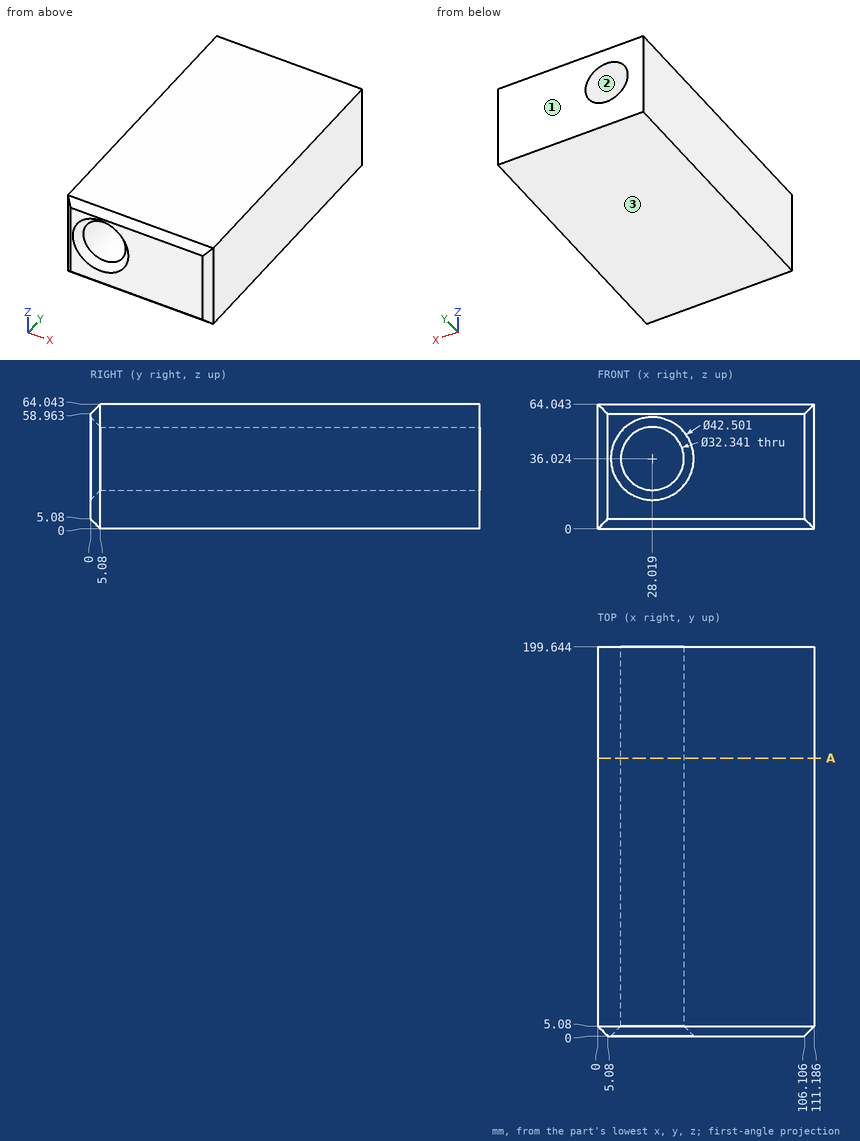
Geometry check sheet. Reference: drawing and pictorial views, mm from the part's lowest x, y, z. Coordinates: 2 decimals unless noted, no trailing zeros. Write each loop counter-clockwise with the first axis right and the second up, starting at its lowest first coordinate (ties: lowest second). Pieces come first, ordered by that corner, then holes. Notation, with made-up numbers: (9.5, 69.25) - (26.5, 69.25) arc R20 cw to (26.5, 98.25) - close; hole circle Ø3 at (50, 28). An arc over 180 degrees is marked (long way). Write item = value, one per line.
Q1. Go/stop test with a flat-tipped pin: pin 1 Ø12 at (x, y) = (59.5, 103.5) entering from -Z. Record where the tip stops, or that it passes through.
Answer:
pin_1 = 0
Q2. Mould release check, pull along Z, two halves, no side actions. Record for the marked faces 1, 2 and 3: released by +Z, released by -Z, zero draft, split by the parting line, or undercut.
Answer:
face_1 = zero draft
face_2 = undercut
face_3 = released by -Z
Q3. Material ranges on L1, parallel to Z at x = 27.5, y = 130; L2, parallel to X at y = 15, z = 35; L3, parallel to X at y = 73, z = 44.5 (1 decimal), recorded low to high. Write a range as from..to.
Answer:
L1 = 0..19.86, 52.19..64.04
L2 = 0..11.88, 44.16..111.19
L3 = 0..14.2, 41.8..111.2
Q4. Cross-section at A-A (y = 142.5). Enter the section's corners in (x, z) (1 decimal).
Answer:
outline = (0, 0) - (111.2, 0) - (111.2, 64) - (0, 64) - close; hole circle Ø32.3 at (28, 36)
